Geometry: final body of the model. Coordinates: model frame, mm. A direction names the side the tool comes from. Give positions to 0.01 mm unless a question says otherwise; leave off trailing zeros. Write each loop counter-clockwise with the first axis right and the second up, starting at its lowest first coordinate (ties: lowest second). Pieces come first, ordered by that corner, then holes. Notation, with made-up numbers: (-3.75, 50) -> (47.25, 50) arc R28 cw to (47.25, 76) -> close; hole circle Ø1 at (21, 52). An arc over 180 degrees is marked (long way). Answer in a Markdown table with one row per item. Add a question column.
Item 1: Material intervals for probe 1 along Z at (x, y) = (8, 1.6); probe 2 along X at (y, z) = (5.75, -8), sorted ascending. Write a range as from..to.
Item 2: Section query D-D on x = 0. Output: boundary loops of the cut face in (y, z).
Item 3: Draft query along X for faces 3 (the flat face through (0, 0, -8)), 4 (the flat face through (-11.55, 3, 0)), 5 (the flat face through (-9, 4.4, 7)). Return one class per face: +X half, -X half, draft (parallel to the pull), parting line (faces both ways), or undercut.
Item 4: Access query for faces 1 (the flat face through (-9, 4.4, -9)), 2 (the flat face through (0, 3, -11.55)). Directions: +Z, -Z, +X, -X, +Y, -Y. A direction counts if a zero-diameter tool reaches every point of the face in a straight line with its end or side. Return the directions, or none.
Item 5: Section query B-B on x = 8. Output: boundary loops of the cut face in (y, z), plus the area to 3 significant figures.
Item 6: Section query A-A on y = 1.5. Output: boundary loops of the cut face in (x, z).
Item 7: First-contact query: P1, Ø2, axis at x = -8, z = -8.5, coming from the +Y side; P2, Ø1.8, axis at x = 8, z = -8, coming from the -Y side. Flat tips, straight axial feed; report the tip coordinate or a pass-through.
Item 8: Section query C-C on y = 3.75. Output: boundary loops of the cut face in (x, z), plus the area to 3 significant figures.
Autodesk Fusion 360 part; units mm, degrees
sketch "Sketch1" plane through (0, 0, 0) normal (0, 1, 0) x (1, 0, 0)
  line L0 (11.55, -11.55) -> (-11.55, -11.55)
  line L1 (-11.55, -11.55) -> (-11.55, 11.55)
  line L2 (-11.55, 11.55) -> (11.55, 11.55)
  line L3 (11.55, 11.55) -> (11.55, -11.55)
  line L4 (11.55, -11.55) -> (-11.55, 11.55) construction
  line L5 (-11.55, -11.55) -> (11.55, 11.55) construction
  dimension "d1" = 23.1
  dimension "d2" = 23.1
extrude "Extrude1" add sketch "Sketch1" along normal blind 6.4
sketch "Sketch2" plane through (0, 6.4, 0) normal (0, 1, 0) x (-1, 0, 0)
  line L0 (-11.55, -11.55) -> (11.55, -11.55)
  line L1 (11.55, -11.55) -> (11.55, 11.55)
  line L2 (11.55, 11.55) -> (-11.55, 11.55)
  line L3 (-11.55, 11.55) -> (-11.55, -11.55)
  line L4 (-8, 8) -> (8, 8) construction
  line L5 (8, 8) -> (8, -8) construction
  line L6 (8, -8) -> (-8, -8) construction
  line L7 (-8, -8) -> (-8, 8) construction
  line L8 (-8, 8) -> (8, -8) construction
  line L9 (8, 8) -> (-8, -8) construction
  circle A0 centre (0, 0) radius 7.6
  point P0 (8, -8)
  point P1 (-8, -8)
  point P2 (-8, 8)
  point P3 (8, 8)
  dimension "d5" = 16
  dimension "d6" = 16
  dimension "d7" = 15.2
hole "Hole1" at (-8, 6.4, -8) direction (0, -1, 0) diameter 2.2 end through all counterbore diameter 4.4 counterbore depth 2
hole "Hole2" at (8, 6.4, -8) direction (0, -1, 0) diameter 2.2 end through all counterbore diameter 4.4 counterbore depth 2
hole "Hole3" at (8, 6.4, 8) direction (0, -1, 0) diameter 2.2 end through all counterbore diameter 4.4 counterbore depth 2
hole "Hole4" at (-8, 6.4, 8) direction (0, -1, 0) diameter 2.2 end through all counterbore diameter 4.4 counterbore depth 2
extrude "Extrude2" cut sketch "Sketch2" along normal through all and the other way through all contours A0
sketch "Sketch3" plane through (0, 0, 11.55) normal (0, 0, 1) x (1, 0, 0)
  line L0 (-11.55, 0) -> (11.55, 0)
  line L1 (11.55, 0) -> (11.55, 6.4)
  line L2 (11.55, 6.4) -> (-11.55, 6.4)
  line L3 (-11.55, 6.4) -> (-11.55, 0)
  line L4 (-11.55, 3.2) -> (11.55, 3.2) construction
  point P0 (-4.15, 3.2)
  point P1 (3.99, 3.2)
  dimension "d29" = 8.14
  dimension "d30" = 7.4
hole "Hole5" at (-4.07, 3.2, 11.55) direction (0, 0, -1) diameter 2.05 depth 7 tip angle 118
hole "Hole6" at (4.07, 3.2, 11.55) direction (0, 0, -1) diameter 2.05 depth 7 tip angle 118
Findings below:
| question | item | result |
|---|---|---|
| 1 | probe 1 | z = -11.55..-9.1, -6.9..6.9, 9.1..11.55 |
| 1 | probe 2 | x = -11.55..-10.2, -5.8..5.8, 10.2..11.55 |
| 2 | outline | (0, -11.55) -> (6.4, -11.55) -> (6.4, -7.6) -> (0, -7.6) -> close; (0, 7.6) -> (6.4, 7.6) -> (6.4, 11.55) -> (0, 11.55) -> close |
| 3 | face 3 | draft |
| 3 | face 4 | -X half |
| 3 | face 5 | undercut |
| 4 | face 1 | +Y |
| 4 | face 2 | -Z, +X, -X, +Y, -Y |
| 5 | outline | (0, -11.55) -> (6.4, -11.55) -> (6.4, -10.2) -> (4.4, -10.2) -> (4.4, -9.1) -> (0, -9.1) -> close; (0, -6.9) -> (4.4, -6.9) -> (4.4, -5.8) -> (6.4, -5.8) -> (6.4, 5.8) -> (4.4, 5.8) -> (4.4, 6.9) -> (0, 6.9) -> close; (0, 9.1) -> (4.4, 9.1) -> (4.4, 10.2) -> (6.4, 10.2) -> (6.4, 11.55) -> (0, 11.55) -> close |
| 5 | area | 111 mm^2 |
| 6 | outline | (-11.55, -11.55) -> (11.55, -11.55) -> (11.55, 11.55) -> (-11.55, 11.55) -> close; hole circle Ø2.2 at (-8, -8); hole circle Ø2.2 at (-8, 8); hole circle Ø15.2 at (0, 0); hole circle Ø2.2 at (8, -8); hole circle Ø2.2 at (8, 8) |
| 7 | P1 | stops at y = 4.4 |
| 7 | P2 | passes through |
| 8 | outline | (-11.55, -11.55) -> (11.55, -11.55) -> (11.55, 11.55) -> (4.93, 11.55) -> (4.93, 5.78) arc R7.6 cw (long way) to (-4.93, 5.78) -> (-4.93, 11.55) -> (-11.55, 11.55) -> close; (-3.21, 6.89) arc R7.6 cw to (3.21, 6.89) -> (3.21, 11.55) -> (-3.21, 11.55) -> close; hole circle Ø2.2 at (-8, -8); hole circle Ø2.2 at (-8, 8); hole circle Ø2.2 at (8, -8); hole circle Ø2.2 at (8, 8) |
| 8 | area | 319 mm^2 |
